Can you work these out from the drawing? Everything is in mm from the part's minimum corner. Round coordinates to 2 decimals unless told otherwise and drop trailing zeros. Write each loop counter-clockwise with the first axis right and the second up, starting at its lowest first coordinate (ties: lowest second). Pieces come first, ordered by that corner, then holes. Notation, with made-up numbers: M 25.25,58.5 L 70.25,58.5 A5 ccw 70.25,65.5 Z; hole C 38,16.25 d5. An arc over 180 degrees is marked long. Answer in a Markdown table with one row per item. Add a question column.
(1) Suppose I cut it at C-C, the plane z = 25.4. Write out the boundary of the cut face in (x, y) (3 decimals).
(2) Suppose I cut it at B-B, the plane y = 2.65. Write out the boundary of the cut face in (x, z) (3 decimals), then the cut area to 3 significant figures.
(3) Suppose I cut it at D-D, the plane x = 228.6. Write out the boundary of the cut face in (y, z) (3 decimals).
(4) I'm going to push a flat-ended pin straight in: pin 1 (1.5 mm diameter, centred on y = 2.5, z = 76.5, fed in from +X) (3 decimals). Where does the tip first touch, or does it pass through?
(5) Suppose I cut it at A-A, the plane x = 127. Write out the boundary of the cut face in (y, z) (3 decimals).
(6) If I drill on probe 1 along Z at (x, y) = (127, 1.3) (3 decimals); probe 2 along Z at (x, y) = (129, 0.25); probe 3 along Z at (x, y) = (226, 2.15), over which ranges is the centre line in solid material (lowest first)?
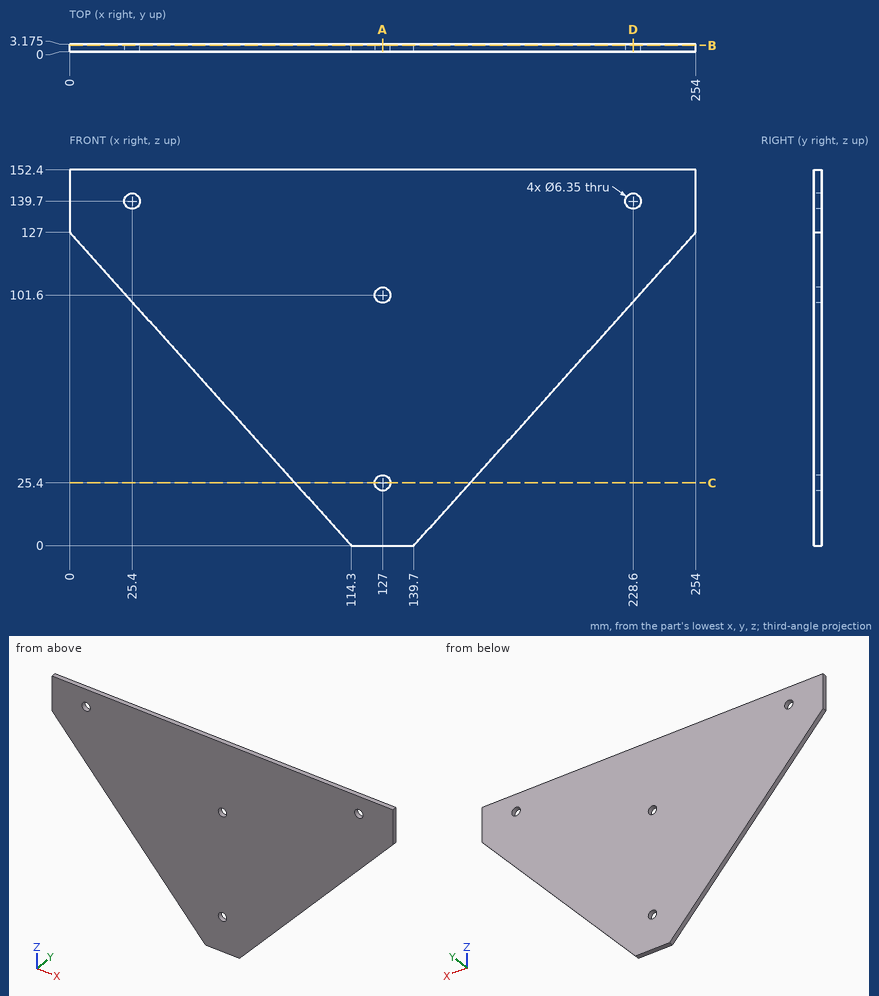
Calculated:
| question | item | result |
|---|---|---|
| 1 | outline | M 91.44,0 L 123.825,0 L 123.825,3.175 L 91.44,3.175 Z; M 130.175,0 L 162.56,0 L 162.56,3.175 L 130.175,3.175 Z |
| 2 | outline | M 0,127 L 114.3,0 L 139.7,0 L 254,127 L 254,152.4 L 0,152.4 Z; hole C 25.4,139.7 d6.35; hole C 127,25.4 d6.35; hole C 127,101.6 d6.35; hole C 228.6,139.7 d6.35 |
| 2 | area | 24,100 mm² |
| 3 | outline | M 0,98.778 L 3.175,98.778 L 3.175,136.525 L 0,136.525 Z; M 0,142.875 L 3.175,142.875 L 3.175,152.4 L 0,152.4 Z |
| 4 | pin 1 | x = 209.225 |
| 5 | outline | M 0,0 L 3.175,0 L 3.175,22.225 L 0,22.225 Z; M 0,28.575 L 3.175,28.575 L 3.175,98.425 L 0,98.425 Z; M 0,104.775 L 3.175,104.775 L 3.175,152.4 L 0,152.4 Z |
| 6 | probe 1 | 0 to 22.225, 28.575 to 98.425, 104.775 to 152.4 |
| 6 | probe 2 | 0 to 22.93, 27.87 to 99.13, 104.07 to 152.4 |
| 6 | probe 3 | 95.89 to 137.88, 141.52 to 152.4 |
